Check sheet for the modelled part. Datum: model origin and axes. Units: mm. A direction names the side the tool comes from. Coordinates: 2 decimals unless noted, no trailing zeros. Order: outer loops, then holes, each group sorted by start corner. A loop starts at its lowest first (then second) coordinate and runs counter-clockwise, first axis right, second up.
from build123d import *

# Parameters (mm, degrees)
EXTRUDE_1_DEPTH      = 5.5
SKETCH_5_R           = 0.75
CUT_EXTRUDE_3_DEPTH  = 135.373546504
SKETCH_6_R           = 1.05
CUT_EXTRUDE_4_DEPTH  = 135.373546504
SKETCH_8_W           = 5.5
SKETCH_8_H           = 5.5
CUT_EXTRUDE_6_DEPTH  = 135.373546504
SKETCH_9_R           = 1.05
CUT_EXTRUDE_7_DEPTH  = 135.373546504
SKETCH_10_W          = 5.5
SKETCH_10_H          = 100
CUT_EXTRUDE_8_DEPTH  = 135.373546504
SKETCH_11_R          = 1.05
CUT_EXTRUDE_9_DEPTH  = 135.373546504
SKETCH_12_R          = 1.05
SKETCH_12_W          = 22.5
SKETCH_12_H          = 12.2
CUT_EXTRUDE_10_DEPTH = 10
FILLET_1_R           = 5
FILLET_2_R           = 5


with BuildPart() as part:
    # ｽｹｯﾁ1 → ﾎﾞｽ - 押し出し1 (new body)
    with BuildSketch(Plane.XY):
        with BuildLine():
            Line((19, 125), (-43, 125))
            Line((-43, 125), (-43, 69))
            Line((-43, 69), (-19, 69))
            Line((-19, 69), (-19, 23.216373532))
            ThreePointArc((-19, 23.216373532), (0, -30), (19, 23.216373532))
            Line((19, 23.216373532), (19, 115))
            Line((19, 115), (49, 115))
            Line((49, 115), (49, 125))
            Line((49, 125), (19, 125))
        make_face()
    extrude(amount=EXTRUDE_1_DEPTH)

    # ｽｹｯﾁ5 → ｶｯﾄ - 押し出し3 (cut, through all)
    with BuildSketch(Plane.XY.offset(5.5)):
        with Locations((14.45, 0)):
            Circle(SKETCH_5_R)
        with Locations((-14.45, 0)):
            Circle(SKETCH_5_R)
    extrude(amount=-CUT_EXTRUDE_3_DEPTH, mode=Mode.SUBTRACT)

    # ｽｹｯﾁ6 → ｶｯﾄ - 押し出し4 (cut, through all)
    with BuildSketch(Plane.XY.offset(5.5)):
        with Locations((-24.425038206, -12.880897043)):
            Circle(SKETCH_6_R)
        with Locations((-21.701843031, -17.074249883)):
            Circle(SKETCH_6_R)
        with Locations(Location((24.425038206, -12.880897043, 0), (0, 0, 180))):
            Circle(SKETCH_6_R)
        with Locations(Location((21.701843031, -17.074249883, 0), (0, 0, 180))):
            Circle(SKETCH_6_R)
    extrude(amount=-CUT_EXTRUDE_4_DEPTH, mode=Mode.SUBTRACT)

    # ｽｹｯﾁ8 → ｶｯﾄ - 押し出し6 (cut, through all)
    with BuildSketch(Plane.XY.offset(5.5)):
        with Locations((12.75, 110.25)):
            Rectangle(SKETCH_8_W, SKETCH_8_H)
        with Locations((-19.75, 110.25)):
            Rectangle(SKETCH_8_W, SKETCH_8_H)
        with Locations((12.75, 77.75)):
            Rectangle(SKETCH_8_W, SKETCH_8_H)
    extrude(amount=-CUT_EXTRUDE_6_DEPTH, mode=Mode.SUBTRACT)

    # ｽｹｯﾁ9 → ｶｯﾄ - 押し出し7 (cut, through all)
    with BuildSketch(Plane.XY.offset(5.5)):
        with Locations((16, 25)):
            Circle(SKETCH_9_R)
        with Locations((16, 29)):
            Circle(SKETCH_9_R)
        with Locations((16, 33)):
            Circle(SKETCH_9_R)
        with Locations((16, 37)):
            Circle(SKETCH_9_R)
        with Locations((16, 41)):
            Circle(SKETCH_9_R)
        with Locations((16, 45)):
            Circle(SKETCH_9_R)
        with Locations((16, 49)):
            Circle(SKETCH_9_R)
        with Locations((16, 53)):
            Circle(SKETCH_9_R)
        with Locations((16, 57)):
            Circle(SKETCH_9_R)
        with Locations(Location((-16, 57, 0), (0, 0, 180))):
            Circle(SKETCH_9_R)
        with Locations(Location((-16, 53, 0), (0, 0, 180))):
            Circle(SKETCH_9_R)
        with Locations(Location((-16, 49, 0), (0, 0, 180))):
            Circle(SKETCH_9_R)
        with Locations(Location((-16, 45, 0), (0, 0, 180))):
            Circle(SKETCH_9_R)
        with Locations(Location((-16, 41, 0), (0, 0, 180))):
            Circle(SKETCH_9_R)
        with Locations(Location((-16, 37, 0), (0, 0, 180))):
            Circle(SKETCH_9_R)
        with Locations(Location((-16, 33, 0), (0, 0, 180))):
            Circle(SKETCH_9_R)
        with Locations(Location((-16, 29, 0), (0, 0, 180))):
            Circle(SKETCH_9_R)
        with Locations(Location((-16, 25, 0), (0, 0, 180))):
            Circle(SKETCH_9_R)
    extrude(amount=-CUT_EXTRUDE_7_DEPTH, mode=Mode.SUBTRACT)

    # ｽｹｯﾁ10 → ｶｯﾄ - 押し出し8 (cut, through all)
    with BuildSketch(Plane.XY.offset(5.5)):
        with Locations((0, 75)):
            Rectangle(SKETCH_10_W, SKETCH_10_H)
    extrude(amount=-CUT_EXTRUDE_8_DEPTH, mode=Mode.SUBTRACT)

    # ｽｹｯﾁ11 → ｶｯﾄ - 押し出し9 (cut, through all)
    with BuildSketch(Plane.XY.offset(5.5)):
        with Locations((-13, 104)):
            Circle(SKETCH_11_R)
        with Locations((-29, 104)):
            Circle(SKETCH_11_R)
        with Locations((-13, 88)):
            Circle(SKETCH_11_R)
        with Locations((-29, 88)):
            Circle(SKETCH_11_R)
    extrude(amount=-CUT_EXTRUDE_9_DEPTH, mode=Mode.SUBTRACT)

    # ｽｹｯﾁ12 → ｶｯﾄ - 押し出し10 (cut)
    with BuildSketch(Plane.XY.offset(5.5)):
        with Locations((-40.1, 79)):
            Circle(SKETCH_12_R)
        with Locations((-12.4, 79)):
            Circle(SKETCH_12_R)
        with Locations((-26.25, 79)):
            Rectangle(SKETCH_12_W, SKETCH_12_H)
    extrude(amount=-CUT_EXTRUDE_10_DEPTH, mode=Mode.SUBTRACT)

    # ﾌｨﾚｯﾄ1
    fillet_1_edges = [part.edges().sort_by_distance(p)[0] for p in [
        (-19, 69, 2.75),
        (-43, 69, 2.75),
    ]]
    fillet(fillet_1_edges, radius=FILLET_1_R)

    # ﾌｨﾚｯﾄ2
    fillet_2_edges = [part.edges().sort_by_distance(p)[0] for p in [
        (19, 115, 2.75),
        (49, 115, 2.75),
    ]]
    fillet(fillet_2_edges, radius=FILLET_2_R)


solid = part.part
(1) Go/stop test with flat-tipped pins: P1, Ø1.9, axis at x = -21.7, y = -17.07, coming from the -Z side; P2, Ø2, axis at y = 1.5, z = 2, coming from the +X side; P3, Ø1.6, axis at x = 12.5, z = 2.5, coming from the -Y side; P4, Ø1, axis at x = -24, z = 1, coming from the -Y side. Record where each tip stops, or that it passes through.
Filled in:
P1: passes through
P2: stops at x = 30
P3: stops at y = -27.62
P4: stops at y = -18.65
(2) Cross-section at B-B (z = 2.75). Count the separate pieces of the cut face and the enclosed holes in it, and give its area (3 significant figures).
Filled in:
separate pieces: 1
enclosed holes: 34
area: 7,150 mm2
(3) Tool access check on faces 1 (the cylindrical face through (20, 113, 3)), 2 (the cylindrical face through (48, 117, 3)), 3 (the flat face through (-19, 44, 3)), 4 (the flat face through (-22.5, 110, 3)). Record the directions out of +Z, -Z, +X, -X, +Y, -Y that give a thin tool (end or side, any length) a straight path to the whole face; none if there is none.
Filled in:
face 1: +Z, -Z, +X
face 2: +Z, -Z, +X, -Y
face 3: +Z, -Z, -X
face 4: +Z, -Z
(4) Cross-section at C-C (y = 9). Enter the section's corners in (x, z).
Filled in:
outline: (-28.62, 0) - (28.62, 0) - (28.62, 5.5) - (-28.62, 5.5) - close
(5) Cross-section at A-A (x = -35.5). Enter the section's corners in (y, z), and give its area (3 significant figures).
Filled in:
outline: (69, 0) - (72.9, 0) - (72.9, 5.5) - (69, 5.5) - close; (85.1, 0) - (125, 0) - (125, 5.5) - (85.1, 5.5) - close
area: 241 mm2
(6) Release check for a two-part mould opening along X. For faces 5 (the cylindrical face through (-21, 68, 3)), 6 (the flat face through (19, 66, 3)), 7 (the flat face through (-37.5, 79, 3)), 8 (the flat face through (34, 115, 3)) record: +X half, -X half, draft (parallel to the pull), parting line (faces both ways), or undercut.
Filled in:
face 5: -X half
face 6: +X half
face 7: undercut
face 8: draft
(7) Thickness scan on probe 1 along X at (y, z) = (79, 1.9); probe 2 along Y at (x, z) = (-26, 4); probe 3 along X at (y, z) = (63, 2). Record the ranges inside material, lowest first.
Filled in:
probe 1: x = -43 to -41.15, -39.05 to -37.5, -15 to -13.45, -11.35 to -2.75, 2.75 to 10, 15.5 to 19
probe 2: y = -14.97 to 14.97, 69 to 72.9, 85.1 to 125
probe 3: x = -19 to -2.75, 2.75 to 19
